```python
from build123d import *

# Parameters (mm, degrees)
SKETCH2_R          = 2.5
CUT_EXTRUDE1_DEPTH = 20


with BuildPart() as part:
    # Sketch1 → Revolve1 (revolve)
    with BuildSketch(Plane.XY, mode=Mode.PRIVATE) as revolve1_sk:
        Polygon((-45.033, 0), (45.033, 0), (45.033, 3.75), (40.033, 3.75), (40.033, 7.5), (-40.033, 7.5), (-40.033, 3.75), (-45.033, 3.75), align=None)
    revolve(revolve1_sk.sketch.rotate(Axis((-45.033, 0, 0), (1, 0, 0)), 180), axis=Axis((-45.033, 0, 0), (1, 0, 0)))

    # Sketch2 → Cut-Extrude1 (cut)
    with BuildSketch(Plane(origin=(45.033, 0, 0), x_dir=(0, 0, -1), z_dir=(1, 0, 0))):
        Circle(SKETCH2_R)
    cut_extrude1 = extrude(amount=-CUT_EXTRUDE1_DEPTH, mode=Mode.SUBTRACT)

    # Mirror1: Cut-Extrude1 across plane
    add(cut_extrude1.mirror(Plane(origin=(0, 0, 0), x_dir=(0, 0, 1), z_dir=(1, 0, 0))), mode=Mode.SUBTRACT)


solid = part.part
```
Model file for the job. Use its own axes, mm. A direction names the side the tool comes from. Coordinates: 2 decimals unless noted, no trailing zeros. Order: outer loops, then holes, each group sorted by start corner. A loop starts at its lowest first (then second) coordinate and runs counter-clockwise, first axis right, second up. Notation, with made-up numbers: (-10.5, 70.25) - (5.5, 70.25) arc R21 ccw to (5.5, 109.25) - close; hole circle Ø4 at (31, 50). An arc over 180 degrees is marked (long way). Return JSON: item names as keys, results as strings. Group by question number.
1) Flat gauge pins, fed straight in: P1, Ø4, axis at y = 0, z = 0, coming from the +X side; P2, Ø3, axis at x = -24, y = 3.5, coming from the +Z side; P3, Ø4, axis at y = 5, z = -4, coming from the +X side. Where does each tip first touch, or does it go through?
2) Probe line 1 (X direction, y = -3.25, z = 4.75); line 2 (Z direction, x = 25.5, y = -2.25); line 3 (Z direction, x = 40.5, y = 1). List the from-to ranges inside material, lowest first. Write a range as from..to.
3) Saw through at A-A, the plane z = 0. Write the cut outline in (x, y).
4) Saw through at D-D, the plane x = -30. Write the cut outline in (y, z), plus the area to 3 significant figures.
5) Tool access for faces 4 (the flat face through (-45.033, 0, -3)), 5 (the flat face through (-25.033, 0, 0)), 6 (the flat face through (25.033, 0, 0)): list every direction of +Z, -Z, +X, -X, +Y, -Y with a clear straight run to the whole face (end or side of a thin tool).
6) Saw through at C-C, the plane x = 8. Write the cut outline in (y, z).
7) Mould opens along Z. For faces 1 (the cylindrical face through (-42.57, -2.02, -3.16)), 2 (the cylindrical face through (-35.17, -2.44, 0.54)), 3 (the flat face through (-40.033, -3, 3)) say: released by +Z, released by -Z, zero draft, split by the parting line, or undercut.
Values found:
{
 "1": {"P1": "stops at x = 25.03", "P2": "stops at z = 7.23", "P3": "stops at x = 40.03"},
 "2": {"line 1": "x = -40.03..40.03", "line 2": "z = -7.15..-1.09, 1.09..7.15", "line 3": "z = -3.61..-2.29, 2.29..3.61"},
 "3": {"outline": "(-45.03, -3.75) - (-40.03, -3.75) - (-40.03, -7.5) - (40.03, -7.5) - (40.03, -3.75) - (45.03, -3.75) - (45.03, -2.5) - (25.03, -2.5) - (25.03, 2.5) - (45.03, 2.5) - (45.03, 3.75) - (40.03, 3.75) - (40.03, 7.5) - (-40.03, 7.5) - (-40.03, 3.75) - (-45.03, 3.75) - (-45.03, 2.5) - (-25.03, 2.5) - (-25.03, -2.5) - (-45.03, -2.5) - close"},
 "4": {"outline": "circle Ø15 at (0, 0); hole circle Ø5 at (0, 0)", "area": "157 mm²"},
 "5": {"face 4": "+Z, -Z, -X, +Y, -Y", "face 5": "-X", "face 6": "+X"},
 "6": {"outline": "circle Ø15 at (0, 0)"},
 "7": {"face 1": "split by the parting line", "face 2": "undercut", "face 3": "zero draft"}
}
